Autodesk Inventor part; units mm, degrees
ref_plane "YZ Plane" through (0, 0, 0) normal (1, 0, 0) x (0, 1, 0)
ref_plane "XZ Plane" through (0, 0, 0) normal (0, 1, 0) x (-1, 0, 0)
ref_plane "XY Plane" through (0, 0, 0) normal (0, 0, 1) x (1, 0, 0)
sketch "Sketch1" plane through (0, 0, 0) normal (0, 0, 1) x (1, 0, 0)
  line L0 (0, 3.7) -> (-2.6393, 3.7)
  line L1 (-2.6393, 3.7) -> (-5.5, 6.5607)
  line L2 (-5.5, 6.5607) -> (-5.5, 8.2)
  line L3 (-5.5, 8.2) -> (-3.395, 8.2)
  line L4 (-3.395, 8.2) -> (-3.395, 10)
  line L5 (-3.395, 10) -> (-10, 10)
  line L6 (-10, 10) -> (-10, 3.395)
  line L7 (-10, 3.395) -> (-8.2, 3.395)
  line L8 (-8.2, 3.395) -> (-8.2, 5.5)
  line L9 (-8.2, 5.5) -> (-6.5607, 5.5)
  line L10 (-6.5607, 5.5) -> (-3.7, 2.6393)
  line L11 (-3.7, 2.6393) -> (-3.7, 0)
  line L12 (0, 0) -> (-10, 10) construction
  circle A0 centre (0, 0) radius 2.3
  line L13 (-12.46, 0) -> (4.76, 0)
  line L14 (-3.7, 0) -> (0, 0)
  line L15 (0, 0) -> (0, 3.7)
  point P0 (-2.3, 0)
  point P1 (0, 2.3)
  dimension "d0" = 1.5
  dimension "d6" = 6.3
  dimension "d9" = 4.6
  dimension "d18" = 135
  dimension "d22" = 20
  dimension "d34" = 11
  dimension "d35" = 6.79
  dimension "d36" = 1.8
extrude "Extrusion1" add sketch "Sketch1" along normal mid plane 300 contours L15 A0 L13 L11 L10 L9 L8 L7 L6 L5 L4 L3 L2 L1 L0
pattern_circular "Circular Pattern1" count 4 over 360 about axis through (0, 0, -10) along (0, 0, 1) of "Extrusion1"
chamfer "Chamfer1" distance 1.185 angle 45 8 edges at (-3.395, 10, 0) (3.395, 10, 0) (10, 3.395, 0) (10, -3.395, 0) (3.395, -10, 0) (-3.395, -10, 0) (-10, -3.395, 0) (-10, 3.395, 0)
fillet "Fillet1" radius 1.5 4 edges at (-10, 10, 0) (10, 10, 0) (-10, -10, 0) (10, -10, 0)
properties part number "2020aluminum_extrusion_silver" material "Aluminum 6061"
Verification items for the finished model (mm, model axes). A direction names the side the tool comes from. Round coordinates to 2 decimals unless told otherwise and drop trailing zeros.
1. Release check for a two-part mould opening along Y. For faces 1 (the flat face through (0, -3.7, -2)), 2 (the flat face through (3.7, 0, -2)), 3 (the flat face through (0, 3.7, -2)) record: +Y half, -Y half, draft (parallel to the pull), parting line (faces both ways), or undercut.
Final values:
face 1: -Y half
face 2: undercut
face 3: +Y half
2. Go/stop test with flat-tipped pins: P1, Ø5, axis at y = -1.5, z = 27, coming from the +X side; P2, Ø1.6, axis at y = -0.5, z = 10, coming from the -X side; P3, Ø6, axis at x = -0.5, z = -14, coming from the +Y side. Record where each tip stops, or that it passes through.
Final values:
P1: stops at x = 9.42
P2: stops at x = -3.7
P3: stops at y = 8.92
3. Access from +Z, -Z, +X, -X, +Y, -Y to the whole of each face (thin tool, end or side, straight path). Record for faces 4 (the flat face through (-2, 2, 150)), 5 (the flat face through (-3.7, 0, -2)).
Final values:
face 4: +Z, +X, -X, +Y, -Y
face 5: +Z, -Z, -X
4. Thickness scan on L1, parallel to Y at x = -7.5, z = -67.5; L2, parallel to X at y = 0, z = 58. Record the ranges inside material, lowest first.
Final values:
L1: y = -10 to -5.5, 5.5 to 10
L2: x = -3.7 to -2.3, 2.3 to 3.7
